Drawing for the job (mm, zero at the part's lowest x, y, z). A direction names the side the tool comes from. Round coordinates to 2 decimals unless told otherwise and drop trailing zeros. Order: outer loops, then holes, each group sorted by start corner. A loop starts at its lowest first (then second) coordinate and runs counter-clockwise, first axis right, second up. Notation, with made-up numbers: (-7, 29) -> (21, 29) arc R14 cw to (21, 35) -> close; hole circle Ø4 at (-8.5, -34). An arc over 180 degrees is marked (long way). Use CSV: the item, a comma, the result in double quotes.
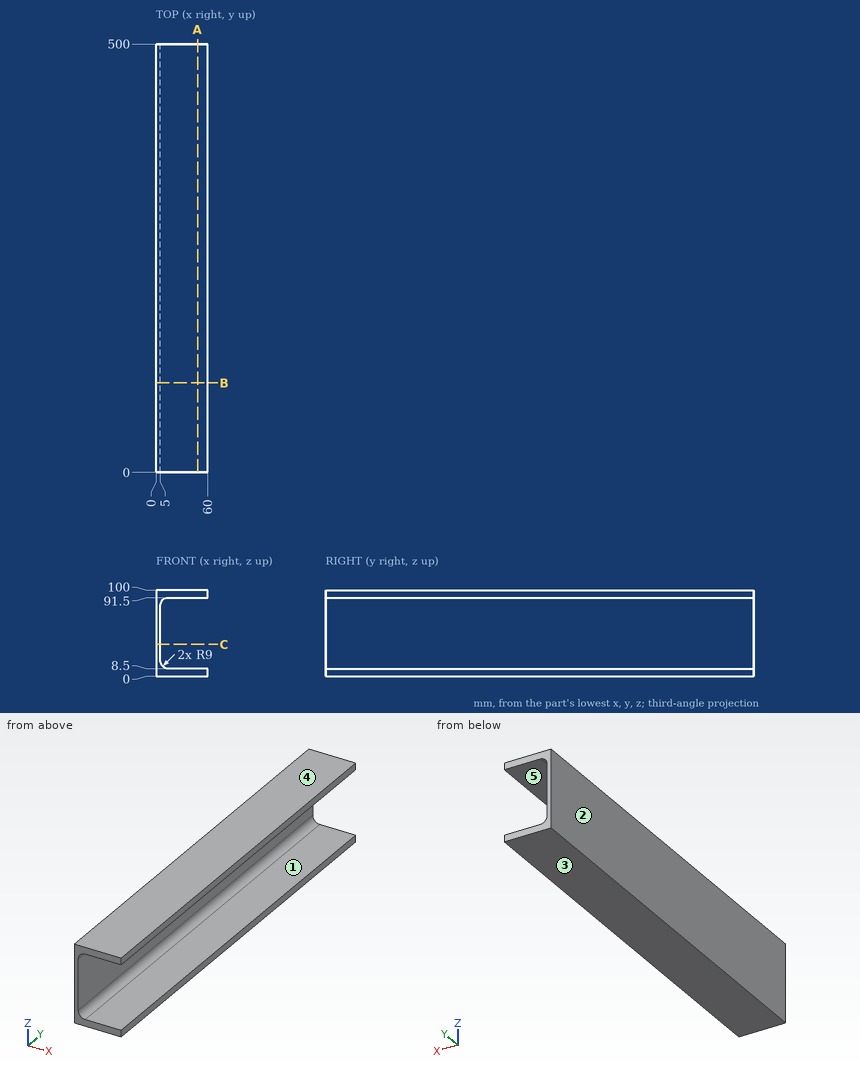
Q1. Which spindle directions (+Z, -Z, +X, -X, +Y, -Y) get a long thin tool onto all of the face, cutting with end or side? Do the marked faces 4 and 5. Say none if no direction does.
From the geometry:
face 4,"+Z, +X, -X, +Y, -Y"
face 5,"+X, +Y, -Y"
Q2. Cut at A-A (x = 48.5). Give the cut face in (y, z).
From the geometry:
outline,"(0, 0) -> (500, 0) -> (500, 8.5) -> (0, 8.5) -> close; (0, 91.5) -> (500, 91.5) -> (500, 100) -> (0, 100) -> close"
Q3. Probe line 1 along Z through (x, y) = (15, 421.5); line 2 along X through (y, z) = (297, 70.5); line 3 along Z through (x, y) = (12.5, 210.5). List the from-to ranges inside material, lowest first.
From the geometry:
line 1,"z = 0 to 8.5, 91.5 to 100"
line 2,"x = 0 to 5"
line 3,"z = 0 to 8.63, 91.37 to 100"
Q4. Cut at C-C (z = 37). Give the cut face in (x, y).
From the geometry:
outline,"(0, 0) -> (5, 0) -> (5, 500) -> (0, 500) -> close"
Q5. Mould opens along Z. For the marked faces 1, 2 and 3 say: +Z half, -Z half, draft (parallel to the pull), parting line (faces both ways), or undercut.
From the geometry:
face 1,"undercut"
face 2,"draft"
face 3,"-Z half"
Q6. Pin check, flat tip, straight feed: pin 1 (2 mm diameter, centred on y = 303.5, z = 68, fed in from +X). Stop position of the tip, or through.
From the geometry:
pin 1,"stops at x = 5"
Q7. Cut at B-B (y = 104.5). Give the cut face in (x, z).
From the geometry:
outline,"(0, 0) -> (60, 0) -> (60, 8.5) -> (14, 8.5) arc R9 cw to (5, 17.5) -> (5, 82.5) arc R9 cw to (14, 91.5) -> (60, 91.5) -> (60, 100) -> (0, 100) -> close"
